The figure shows three views and two pictorial views of one solid part (mm, origin at its lowest corner). Answer the questions. A direction names the side the tool comes from. Give positions to 0.01 mm unless a question says otherwise; leave off trailing zeros. Write each loop counter-clockwise with the first axis right and the second up, starting at its lowest first coordinate (ties: lowest second). Pieces come first, ordered by that corner, then holes. Notation, with made-up numbers: (53.5, -25.5) -> (87.5, -25.5) arc R19 ccw to (87.5, 7.5) -> close; hole circle Ø6 at (47, -33). An arc over 180 degrees is marked (long way). Use a Markdown table: item, result.
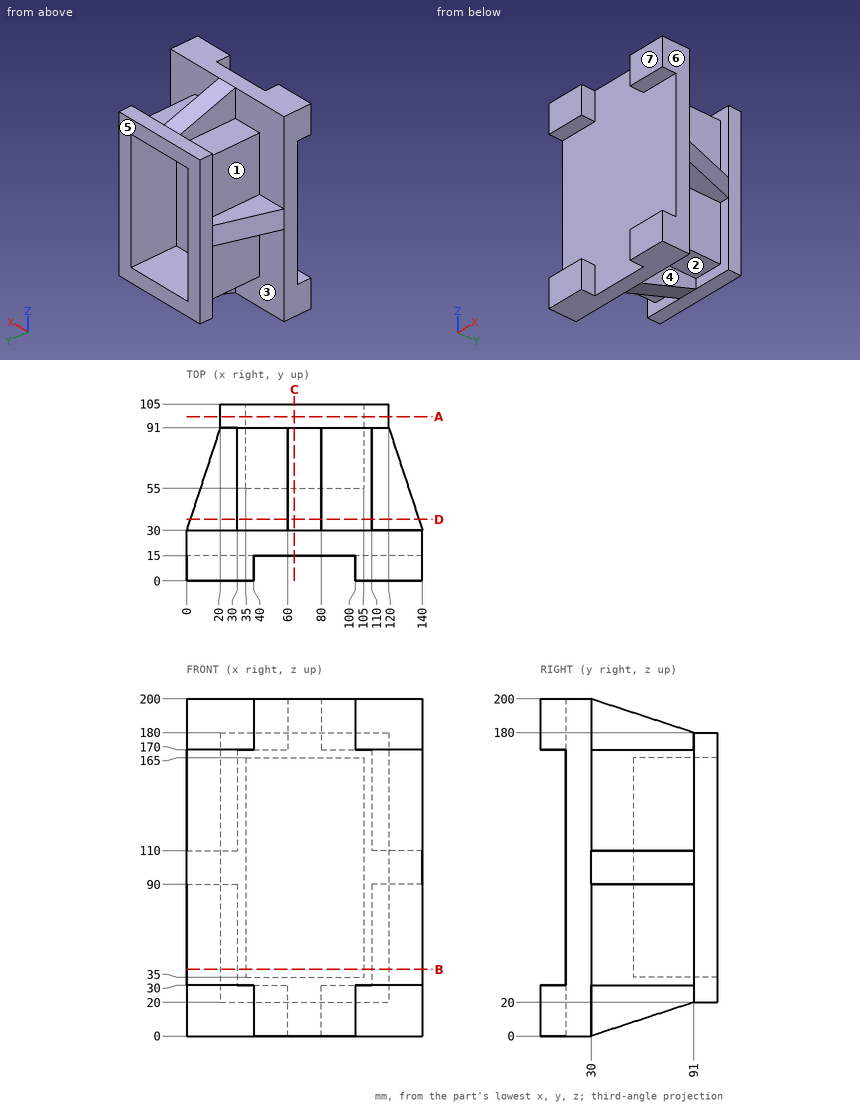
Item 1: For a pull along Y with two mould halves and no side action, classify the marked faces 4, 5, 6 and 7 as +Y half, -Y half, draft (parallel to the pull), parting line (faces both ways), or undercut.
Return value:
| item | result |
|---|---|
| face 4 | undercut |
| face 5 | +Y half |
| face 6 | draft |
| face 7 | -Y half |
Item 2: A cutting plane is placed at A-A (y = 97.5). Give the vertices of the cut face in (x, z), then the cut area to 3 significant figures.
Return value:
| item | result |
|---|---|
| outline | (20, 20) -> (120, 20) -> (120, 180) -> (20, 180) -> close; hole (35, 35) -> (105, 35) -> (105, 165) -> (35, 165) -> close |
| area | 6,900 mm^2 |
Item 3: Straight lines are drawn through the part: line 1 along Z through (x, y) = (98, 90.5); line 2 along Y through (x, z) = (37.5, 171); line 3 along X through (y, z) = (88, 67). For each, find the intervals that lie inside material, in ascending order. Write a range as [from, to].
Return value:
| item | result |
|---|---|
| line 1 | [30, 35], [165, 170] |
| line 2 | [0, 30], [91, 105] |
| line 3 | [30, 35], [105, 110] |
Item 4: A tool of negligible diameter and unlimited length cuts with its end or side. For the marked faces 1, 2 and 3, from which of +Z, -Z, +X, -X, +Y, -Y can it reach the whole face along a straight path? Write none if from no direction.
Return value:
| item | result |
|---|---|
| face 1 | +Z, -X |
| face 2 | -Z, +X |
| face 3 | -Z, -X |
Item 5: A cutting plane is placed at D-D (y = 36.5). Give the vertices of the cut face in (x, z), then the cut area to 3 significant figures.
Return value:
| item | result |
|---|---|
| outline | (2.13, 90) -> (30, 90) -> (30, 30) -> (60, 30) -> (60, 2.13) -> (80, 2.13) -> (80, 30) -> (110, 30) -> (110, 90) -> (137.87, 90) -> (137.87, 110) -> (110, 110) -> (110, 170) -> (80, 170) -> (80, 197.87) -> (60, 197.87) -> (60, 170) -> (30, 170) -> (30, 110) -> (2.13, 110) -> close |
| area | 13,400 mm^2 |
Item 6: A cutting plane is placed at B-B (z = 39.5). Give the vertices of the cut face in (x, y).
Return value:
| item | result |
|---|---|
| outline | (0, 15) -> (140, 15) -> (140, 30) -> (110, 30) -> (110, 91) -> (120, 91) -> (120, 105) -> (105, 105) -> (105, 55) -> (35, 55) -> (35, 105) -> (20, 105) -> (20, 91) -> (30, 91) -> (30, 30) -> (0, 30) -> close |
Item 7: Each of these flat-tipped pins is pushed along its axis until it touches: P1, Ø5, axis at x = 38.5, z = 41, coming from the +Y side; P2, Ø10, axis at y = 81.5, z = 135.5, coming from the -X side; P3, Ø24, axis at x = 39.5, y = 63.5, coming from the +Z side; P4, Ø6, axis at x = 125, y = 90.5, coming from the +Z side. Where does it stop, or does it pass through?
Return value:
| item | result |
|---|---|
| P1 | y = 55 |
| P2 | x = 30 |
| P3 | z = 170 |
| P4 | through |
Item 8: A cutting plane is placed at C-C (x = 64). Give the vertices of the cut face in (y, z), then the cut area to 3 significant figures.
Return value:
| item | result |
|---|---|
| outline | (15, 0) -> (30, 0) -> (91, 20) -> (105, 20) -> (105, 35) -> (55, 35) -> (55, 165) -> (105, 165) -> (105, 180) -> (91, 180) -> (30, 200) -> (15, 200) -> close |
| area | 9,720 mm^2 |
